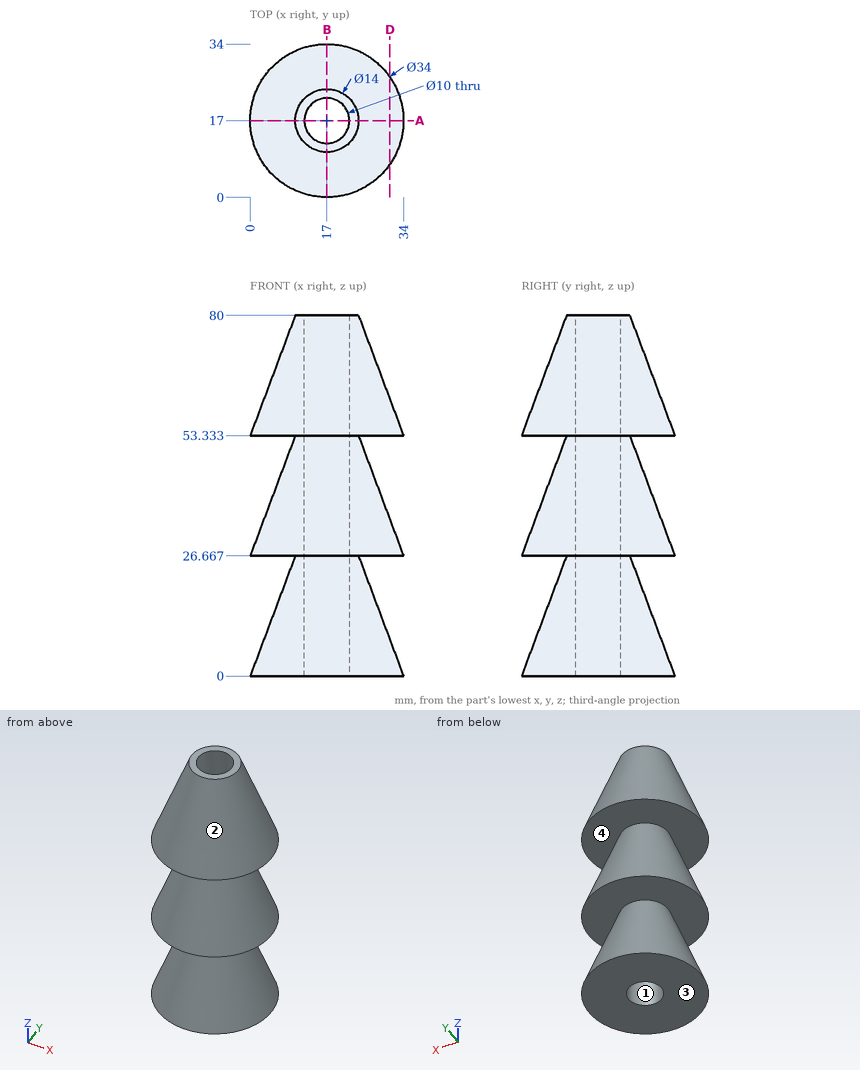
Design review of the part shown in the three views and the two pictorial views. Dimensions are in mm from the part's minimum x, y and z. Round coordinates to 2 decimals unless told otherwise and drop trailing zeros. Loops run counter-clockwise (first coordinate to the right, second up) from the corner with the lowest first, then second, coordinate; pieces in that order, holes last.
Q1. Mouldability with a two-part tool opening along Z and no side actions: class the marked faces 1, 2, 3 and 4 as +Z half, -Z half, draft (parallel to the pull), parting line (faces both ways), or undercut.
Result sheet:
face 1: draft
face 2: +Z half
face 3: -Z half
face 4: undercut
Q2. To check wall thickness, follow line 1 along Z through (x, y) = (31.5, 8.5) (1 decimal); line 2 along Z through (x, y) = (26, 4) (1 decimal); line 3 along Y through (x, z) = (17, 46). State the ranges of each line that lie inside material, in increasing order.
Result sheet:
line 1: z = 0 to 0.5, 26.7 to 27.2, 53.3 to 53.8
line 2: z = 0 to 3.2, 26.7 to 29.8, 53.3 to 56.5
line 3: y = 7.25 to 12, 22 to 26.75
Q3. Insertion check: pin 1 Ø12 at (x, z) = (28.5, 67.5) entering from -Y (1 decimal); pin 2 Ø8 at (y, z) = (17.5, 71) entering from -X; pin 3 Ø12 at (x, z) = (17.5, 14.5) entering from +Y. Each pin has a flat end and moves straight along its axis. Give the tip position at first contact, or say it passes through.
Result sheet:
pin 1: stops at y = 5.8
pin 2: stops at x = 5.13
pin 3: stops at y = 30.81
Q4. Add section D-D on x = 31. Give the number of separate pieces and of enclosed holes in the cut face.
Result sheet:
separate pieces: 3
enclosed holes: 0
Q5. Add section A-A on y = 17. Write out the cut boundary in (x, z), plus the area to 3 significant figures.
Result sheet:
outline: (0, 0) - (12, 0) - (12, 80) - (10, 80) - (0, 53.33) - (10, 53.33) - (0, 26.67) - (10, 26.67) - close; (22, 0) - (34, 0) - (24, 26.67) - (34, 26.67) - (24, 53.33) - (34, 53.33) - (24, 80) - (22, 80) - close
area: 1,120 mm2
